from build123d import *

# Parameters (mm, degrees)
F0_R     = 25
F1_DEPTH = 20
F3_R     = 5
F4_DEPTH = 70


with BuildPart() as f1:
    # F0 (on Front) → F1 (new body)
    with BuildSketch(Plane.XZ):
        with BuildLine():
            Line((-25.191063, 440.046496), (-25.191063, -86.412484))
            Line((-25.191063, -86.412484), (24.808937, -86.412484))
            Line((24.808937, -86.412484), (24.808937, 440.046496))
            ThreePointArc((24.808937, 440.046496), (25.589393, 443.919479), (27.808937, 447.187924))
            ThreePointArc((27.808937, 447.187924), (-0.191063, 515.753638), (-28.191063, 447.187924))
            ThreePointArc((-28.191063, 447.187924), (-25.971518, 443.919479), (-25.191063, 440.046496))
        make_face()
        with Locations((-0.191063, 475.753638)):
            Circle(F0_R, mode=Mode.SUBTRACT)
    extrude(amount=F1_DEPTH)

    # F3
    f3_edges = [f1.edges().sort_by_distance(p)[0] for p in [
        (-25.191063, -20, 176.817006),
        (-25.191063, 0, 176.817006),
    ]]
    fillet(f3_edges, radius=F3_R)

    # F2 (on face) → F4 (cut, symmetric)
    with BuildSketch(Plane(origin=(-25.191063, 0, 0), x_dir=(0, -1, 0), z_dir=(-1, 0, 0))):
        Polygon((7.5, 443.61721), (7.5, 515.753638), (0, 515.753638), (0, 500.753638), (0, 450.753638), (0, 447.187924), (0, 443.61721), align=None)
        Polygon((20, 450.753638), (20, 500.753638), (20, 515.753638), (12.5, 515.753638), (12.5, 443.61721), (20, 443.61721), (20, 447.187924), align=None)
    extrude(amount=F4_DEPTH, both=True, mode=Mode.SUBTRACT)


solid = f1.part
Model file for the job. Use its own axes, mm. A direction names the side the tool comes from. Give positions to 0.01 mm unless a question says otherwise; leave off trailing zeros. Write each loop counter-clockwise with the first axis right and the second up, starting at its lowest first coordinate (ties: lowest second). Pieces come first, ordered by that corner, then holes. Notation, with made-up numbers: (30.5, 39) -> (57.5, 39) arc R12 cw to (57.5, 60) -> close; hole circle Ø7 at (-26, -24). An arc over 180 degrees is marked (long way). Write item = value, one per line.
(1) Probe line 1 along Y through (x, z) = (20, 139); line 2 along Z through (x, y) = (5, -14.75); line 3 along X through (y, z) = (-13.75, 222.5). List the from-to ranges inside material, lowest first.
Determined:
line_1 = -20 to 0
line_2 = -86.41 to 443.62
line_3 = -25.19 to 24.81
(2) Slice it at A-A, the plane x = -7. Give the cut face in (y, z).
Determined:
outline = (-20, -86.41) -> (0, -86.41) -> (0, 443.62) -> (-7.5, 443.62) -> (-7.5, 451.7) -> (-12.5, 451.7) -> (-12.5, 443.62) -> (-20, 443.62) -> close; (-12.5, 499.81) -> (-7.5, 499.81) -> (-7.5, 515.17) -> (-12.5, 515.17) -> close
(3) Tool access for faces 4 (the face through (-19, -12.5, 496)), 5 (the face through (-25.191, -10, 181)), 6 (the face through (-1, -10, -86.412)): list every direction of +Z, -Z, +X, -X, +Y, -Y with a clear straight run to the whole face (end or side of a thin tool).
Determined:
face_4 = +Z, +X, -X, -Y
face_5 = -Z, -X, +Y, -Y
face_6 = -Z, +X, -X, +Y, -Y
(4) Mould opens along Y. For faces 1 (the face through (18, -7.5, 495)), 2 (the face through (0, -20, 182)), 3 (the face through (24.809, -10, 173)) say: released by +Y, released by -Y, zero draft, split by the parting line, or undercut.
Determined:
face_1 = released by +Y
face_2 = released by -Y
face_3 = zero draft
(5) Slice it at B-B, the plane z = 156. Give the cut face in (x, y), then the cut area to 3 significant figures.
Determined:
outline = (-25.19, -15) arc R5 ccw to (-20.19, -20) -> (19.81, -20) arc R5 ccw to (24.81, -15) -> (24.81, -5) arc R5 ccw to (19.81, 0) -> (-20.19, 0) arc R5 ccw to (-25.19, -5) -> close
area = 979 mm2
(6) Flat gauge pins, fed straight in: P1, Ø2.5, axis at x = 0.5, y = -15.5, coming from the +Z side; P2, Ø11, axis at y = -10, z = 124.5, coming from the -X side; P3, Ø1, axis at y = -7, z = 244.5, coming from the +X side; P4, Ø10, axis at x = -22.5, z = 193.5, coming from the +Y side. Where does each tip first touch, or does it go through?
Determined:
P1 = 443.62
P2 = -25.19
P3 = 24.81
P4 = 0
